from build123d import *

# Parameters (mm, degrees)
SUPERFICIE_EXTRUIR1_2_DEPTH = 100
DAR_ESPESOR1_T2             = 2
CROQUIS4_R                  = 37.5
CROQUIS4_R_2                = 4
EXTRUIR3_DEPTH              = 11


with BuildPart() as body_1:
    # Superficie-Extruir1: a surface, the sketch's curves swept straight by 100 mm
    with BuildLine(Plane.XY, mode=Mode.PRIVATE) as superficie_extruir1_2_path:
        Line((-100, -200), (-100, -70))
        ThreePointArc((-100, -70), (-79.497474683, -20.502525317), (-30, 0))
        Line((-30, 0), (0, 0))
        Line((0, 0), (0, -200))
    superficie_extruir1_2 = Shell.extrude(superficie_extruir1_2_path.wire(), (0 * SUPERFICIE_EXTRUIR1_2_DEPTH, 0 * SUPERFICIE_EXTRUIR1_2_DEPTH, 1 * SUPERFICIE_EXTRUIR1_2_DEPTH))
    # Croquis5 → Superficie-Plano1: a flat surface bounded by the sketch
    with BuildSketch(Plane(origin=(0, 0, 100), x_dir=(-1, 0, 0), z_dir=(0, 0, -1)), mode=Mode.PRIVATE) as superficie_plano1_3_region:
        with BuildLine():
            Line((100, -200), (0, -200))
            Line((0, -200), (0, 0))
            Line((0, 0), (30, 0))
            ThreePointArc((30, 0), (79.497474683, -20.502525317), (100, -70))
            Line((100, -70), (100, -200))
        make_face()
    superficie_plano1_3 = superficie_plano1_3_region.sketch.faces()[0]
    # Croquis6 → Superficie-Plano2: a flat surface bounded by the sketch
    with BuildSketch(Plane(origin=(0, 0, 0), x_dir=(-1, 0, 0), z_dir=(0, 0, -1)), mode=Mode.PRIVATE) as superficie_plano2_4_region:
        with BuildLine():
            Line((0, -200), (100, -200))
            Line((100, -200), (100, -70))
            ThreePointArc((100, -70), (79.497474683, -20.502525317), (30, 0))
            Line((30, 0), (0, 0))
            Line((0, 0), (0, -200))
        make_face()
    superficie_plano2_4 = superficie_plano2_4_region.sketch.faces()[0]
    # Superficie-Coser1: the surfaces knitted into one
    superficie_coser1_1 = Shell(Face.sew_faces(superficie_extruir1_2.faces() + superficie_plano1_3.faces() + superficie_plano2_4.faces())[0])
    add(Solid.thicken(superficie_coser1_1, -DAR_ESPESOR1_T2))

    # Croquis4 → Extruir3 (cut)
    with BuildSketch(Plane(origin=(0, 0, 0), x_dir=(0, 0, -1), z_dir=(1, 0, 0))):
        with Locations(Location((-50, -50, 0), (0, 0, 90))):
            Circle(CROQUIS4_R)
        with Locations(Location((-90, -10, 0), (0, 0, 90))):
            Circle(CROQUIS4_R_2)
        with Locations(Location((-10, -10, 0), (0, 0, 90))):
            Circle(CROQUIS4_R_2)
        with Locations(Location((-10, -90, 0), (0, 0, 90))):
            Circle(CROQUIS4_R_2)
        with Locations(Location((-90, -90, 0), (0, 0, 90))):
            Circle(CROQUIS4_R_2)
    extrude(amount=-EXTRUIR3_DEPTH, mode=Mode.SUBTRACT)


solid = body_1.part
CAD build for the part. Positions are in the model's coordinates, mm. A direction names the side the tool comes from. Round coordinates to 2 decimals unless told otherwise and drop trailing zeros. Write each loop counter-clockwise with the first axis right and the second up, starting at its lowest first coordinate (ties: lowest second). Pieces come first, ordered by that corner, then holes.
(1) Drop flat-ended pins along their axis: P1, Ø8, axis at x = -84.5, z = 88, coming from the +Y side; P2, Ø1, axis at x = -50.5, z = 27.5, coming from the +Y side; P3, Ø12, axis at x = -57, z = 24.5, coming from the +Y side. Give the stop position or say it passes through.
(2) Slice it at D-D, the plane y = -148. Write the cut outline in (x, z), and give its area (3 significant figures).
(3) Mould opens along Y. For faces 1 (the face through (0, -121, 49)), 2 (the face through (-16, -2, 49)), 3 (the face through (-0.986, -90.867, 86.095)) say: pulls with the +Y half, pulls with the -Y half, needs draft (parallel to the pull), parting line crosses it, or undercut.
(4) Slice it at A-A, the plane y = -90. Write the cut outline in (x, z).
(5) 3-axis set-ups, long thin cutter, end or side, ignore diameter. For faces 4 (the face through (-100, -136, 49)), 5 (the face through (-0.99, -32.7, 16.73)), 6 (the face through (-51, -100, 98)): which of +Z, -Z, +X, -X, +Y, -Y reach the whole face in a straight line?
(6) Slice it at C-C, the plane z = 27.5. Write the cut outline in (x, y), and give its area (3 significant figures).
(7) Slice it at B-B, the plane z = 10. Write the cut outline in (x, y).
(8) Probe line 1 along Z through (x, y) = (-1.3, -10); line 2 along X through (y, z) = (-178, 17); line 3 along Z through (x, y) = (-66.5, -151). List the from-to ranges inside material, lowest first.
From the geometry:
1. P1: stops at y = -21.53
1. P2: stops at y = -2.92
1. P3: stops at y = -3.22
2. outline: (-100, 0) - (0, 0) - (0, 100) - (-100, 100) - close; hole (-98, 2) - (-2, 2) - (-2, 98) - (-98, 98) - close
2. area: 784 mm2
3. face 1: needs draft
3. face 2: pulls with the -Y half
3. face 3: undercut
4. outline: (-100, 0) - (0, 0) - (0, 6) - (-2, 6) - (-2, 2) - (-98, 2) - (-98, 98) - (-2, 98) - (-2, 94) - (0, 94) - (0, 100) - (-100, 100) - close; (-2, 14) - (0, 14) - (0, 86) - (-2, 86) - close
5. face 4: +Z, -Z, -X, +Y, -Y
5. face 5: +X
5. face 6: -Y
6. outline: (-100, -200) - (-98, -200) - (-98, -70) arc R68 cw to (-30, -2) - (-2, -2) - (-2, -20) - (0, -20) - (0, 0) - (-30, 0) arc R70 ccw to (-100, -70) - close; (-2, -200) - (0, -200) - (0, -80) - (-2, -80) - close
6. area: 813 mm2
7. outline: (-100, -200) - (-98, -200) - (-98, -70) arc R68 cw to (-30, -2) - (-2, -2) - (-2, -6) - (0, -6) - (0, 0) - (-30, 0) arc R70 ccw to (-100, -70) - close; (-2, -200) - (0, -200) - (0, -94) - (-2, -94) - close; (-2, -86) - (0, -86) - (0, -14) - (-2, -14) - close
8. line 1: z = 0 to 6, 14 to 86, 94 to 100
8. line 2: x = -100 to -98, -2 to 0
8. line 3: z = 0 to 2, 98 to 100
